Check sheet for the modelled part. Datum: model origin and axes. Units: mm. Face numbers are marked on the shaded views. A direction names the side the tool comes from. Coordinates: 2 decimals unless noted, no trailing zeros. Loops run counter-clockwise (first coordinate to the right, second up) from the corner with the lowest first, then second, coordinate; pieces in that order, holes last. Notation, with made-up numbers: M -28.5,62 L -18.5,62 A7 cw -18.5,66 Z; hole C 74.25,67 d7. An arc over 180 degrees is marked long. Return JSON: item names as keys, results as strings.
Autodesk Inventor part; units mm, degrees
ref_plane "YZ Plane" through (0, 0, 0) normal (1, 0, 0) x (0, 1, 0)
ref_plane "XZ Plane" through (0, 0, 0) normal (0, 1, 0) x (-1, 0, 0)
ref_plane "XY Plane" through (0, 0, 0) normal (0, 0, 1) x (1, 0, 0)
sketch "Sketch1" plane through (0, 0, 0) normal (0, 0, 1) x (1, 0, 0)
  point P0 (0, 0)
sketch "Sketch2" plane through (0, 0, 0) normal (0, 1, 0) x (-1, 0, 0)
  line L0 (0, 0) -> (0, -22)
  line L1 (0, -22) -> (10, -22)
  line L2 (10, -22) -> (10, 0)
  line L3 (10, 0) -> (0, 0)
  dimension "d0" = 22
  dimension "d1" = 10
extrude "Extrusion1" add sketch "Sketch2" along normal blind 15
sketch "Sketch5" plane through (0, 0, 0) normal (1, 0, 0) x (0, 0, -1)
  line L0 (0, 0) -> (22, 0)
  line L1 (22, 0) -> (22, 15)
  line L2 (0, 15) -> (22, 15)
  line L3 (0, 0) -> (0, 15)
  line L4 (22, 15) -> (0, 15)
  line L5 (0, 15) -> (3, 15)
  line L6 (22, 15) -> (19, 15)
  line L7 (22, 0) -> (0, 0)
  line L8 (11, 0) -> (11, 3)
  line L9 (3, 15) -> (3, 9)
  line L10 (3, 9) -> (19, 9)
  line L11 (19, 9) -> (19, 15)
  arc A0 (3, 9) -> (19, 9) centre (11, 11.3333) ccw
  dimension "d4" = 3
  dimension "d5" = 3
  dimension "d7" = 3
  dimension "d8" = 6
extrude "Extrusion2" cut sketch "Sketch5" against normal blind 17 contours A0 L10 | L2 L11 L10 L9
sketch "Sketch6" plane through (-10, 0, 0) normal (0, 0, 1) x (1, 0, 0)
  line L0 (0, 0) -> (10, 0)
  line L1 (10, 0) -> (10, 15)
  line L2 (0, 15) -> (10, 15)
  line L3 (0, 0) -> (0, 15)
  line L4 (0, 15) -> (10, 15)
  line L5 (5, 15) -> (5, 10.5)
  circle A0 centre (5, 10.5) radius 3.25
  dimension "d11" = 4.5
  dimension "d30" = 6.5
extrude "Extrusion3" cut sketch "Sketch6" against normal blind 31.25 contours A0
sketch "Sketch7" plane through (0, 0, 0) normal (0, -1, 0) x (1, 0, 0)
  line L0 (0, -22) -> (-10, -22)
  line L1 (0, 0) -> (0, -22)
  line L2 (-10, 0) -> (0, 0)
  line L3 (-10, -22) -> (-10, 0)
  line L4 (0, -3) -> (0, -19)
  circle A0 centre (-5, -11) radius 6
  dimension "d15" = 12
extrude "Extrusion4" add sketch "Sketch7" along normal blind 3 contours A0 L3 | L3 A0 L1 | L1 A0
sketch "Sketch8" plane through (-5, -3, -11) normal (0, -1, 0) x (1, 0, 0)
  circle A0 centre (0, 0) radius 6
  circle A1 centre (0, 0) radius 4
  point P0 (5, 11)
  dimension "d18" = 8
extrude "Extrusion5" add sketch "Sketch8" along normal blind 4 contours A1
fillet "Fillet1" radius 28 1 edges at (-9, -3, -11)
sketch "Sketch11" plane through (-5, -7, -11) normal (0, -1, 0) x (1, 0, 0)
  circle A0 centre (0, 0) radius 4
  point P0 (5, 11)
extrude "Extrusion6" add sketch "Sketch11" along normal blind 15
sketch "Sketch12" plane through (-5, -22, -11) normal (0, -1, 0) x (1, 0, 0)
  circle A0 centre (0, 0) radius 3
  point P0 (5, 11)
  dimension "d24" = 6
extrude "Extrusion7" add sketch "Sketch12" along normal blind 3
sketch "Sketch13" plane through (-5, -25, -11) normal (0, -1, 0) x (1, 0, 0)
  circle A0 centre (0, 0) radius 4
  point P0 (5, 11)
extrude "Extrusion8" add sketch "Sketch13" along normal blind 2
fillet "Fillet2" radius 0.25 1 edges at (-8, -22, -11)
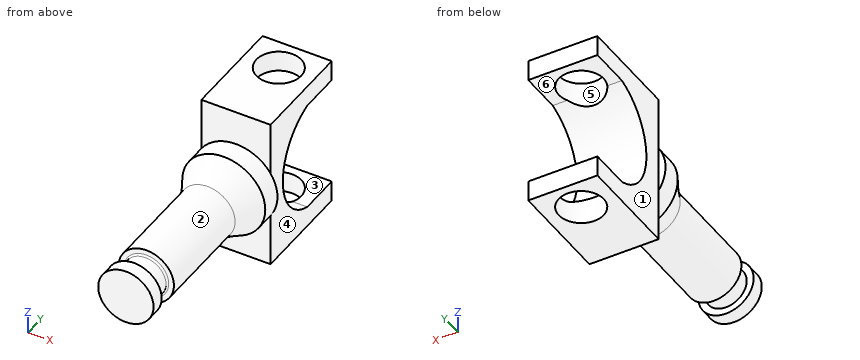
1) Draft check along X on the marked faces 4, 5 and 6. Enter one of: +X half, -X half, draft (parallel to the pull), parting line (faces both ways), or undercut.
Answers:
{"face 4": "+X half", "face 5": "undercut", "face 6": "draft"}
2) Section check A-A on x = -5. Count the separate pieces of the cut face and the enclosed holes in it, then the cut area to 3 significant figures.
Answers:
{"separate pieces": "3", "enclosed holes": "0", "area": "353 mm²"}
3) Section check D-D on z = -11. Record the cut outline in (x, y), then the cut area to 3 significant figures.
Answers:
{"outline": "M -11,-3 A28 cw -9,-7 L -9,-22 L -8.25,-22 A0.25 cw -8,-22.25 L -8,-25 L -9,-25 L -9,-27 L -1,-27 L -1,-25 L -2,-25 L -2,-22.25 A0.25 cw -1.75,-22 L -1,-22 L -1,-7 A28 cw 1,-3 L 1,0 L 0,0 L 0,3 L -10,3 L -10,0 L -11,0 Z", "area": "259 mm²"}
4) Go/stop test with flat-tipped pins: pin 1 Ø1.1 at (x, z) = (0.5, -11.5) entering from +Y; pin 2 Ø5 at (x, y) = (-3.5, 11) entering from +Z; pin 3 Ø3 at (y, z) = (5.5, -7.5) entering from -X; pin 4 Ø12 at (y, z) = (7.5, -14) entering from +X. Record where each tip stops, or that it passes through.
Answers:
{"pin 1": "y = 3.03", "pin 2": "z = 0", "pin 3": "through", "pin 4": "x = 0"}
5) Scan lines: line 1 along Y through (x, z) = (-5, -1.7); line 2 along X through (y, z) = (10.5, -2.7); line 3 along Z through (x, y) = (-9.25, 13). Record each from-to range of solid material in increasing order. Write a range as [from, to].
Answers:
{"line 1": "[0, 7.25], [13.75, 15]", "line 2": "[-10, -8.25], [-1.75, 0]", "line 3": "[-22, -19], [-3, 0]"}
6) Set-up check for the marked faces 1, 2 and 3: record each of +Z, -Z, +X, -X, +Y, -Y from which the full face is reachable in a straight line by a thin tool's end or side.
Answers:
{"face 1": "+Z, -Z, -X, +Y", "face 2": "-Y", "face 3": "+X, -X, +Y"}
7) Section check B-B on y = 10.5. Record the cut outline in (x, z).
Answers:
{"outline": "M -10,-22 L -8.25,-22 L -8.25,-19 L -10,-19 Z; M -10,-3 L -8.25,-3 L -8.25,0 L -10,0 Z; M -1.75,-22 L 0,-22 L 0,-19 L -1.75,-19 Z; M -1.75,-3 L 0,-3 L 0,0 L -1.75,0 Z"}
8) Section check C-C on z = -20.5. Record the cut outline in (x, y), then the cut area to 3 significant figures.
Answers:
{"outline": "M -10,0 L 0,0 L 0,15 L -10,15 Z; hole C -5,10.5 d6.5", "area": "117 mm²"}
